```python
from build123d import *

# Parameters (mm, degrees)
BOSS_EXTRUDE1_START     = -2.5
BOSS_EXTRUDE1_OUTLINE_R = 2.075
BOSS_EXTRUDE1_DEPTH     = 5
FILLET1_R               = 10
FILLET2_R               = 2
SKETCH6_R               = 2.6
CUT_EXTRUDE3_DEPTH      = 0.6
CUT_EXTRUDE4_START      = -0.6
SKETCH7_R               = 2.6
CUT_EXTRUDE4_DEPTH      = 0.6


# Read off the part's stored shape, not the designer's step: Boss-Extrude1
with BuildPart() as part:
    # Boss-Extrude1 outline → Boss-Extrude1 (new body)
    with BuildSketch(Plane(origin=(0, 0, 0), x_dir=(0, 0, -1), z_dir=(1, 0, 0)).offset(BOSS_EXTRUDE1_START)):
        with BuildLine():
            add(Edge.make_bspline(
                [(-11.467759302, 5.348193827), (-9.897325632, 4.539306529), (-6.914913615, 3.521436488), (-2.263899905, 2.426855128), (2.06634335, 1.307705864), (6.2118215, -0.350082751), (10.140310372, -2.114581028), (13.169191833, -3.310542475), (14.923737301, -3.829233653), (15.372310037, -3.948537134)],
                knots=[0.083247791, 0.083247791, 0.083247791, 0.083247791, 0.25, 0.375, 0.5, 0.625, 0.75, 0.875, 0.917679059, 0.917679059, 0.917679059, 0.917679059], degree=3))
            ThreePointArc((-11.467759302, 5.348193827), (-17.179981816, 7.278246829), (-12.961908872, 2.969830498))
            add(Edge.make_bspline(
                [(-12.961908872, 2.969830498), (-12.439456061, 2.692527792), (-10.540790951, 1.792456097), (-7.150824595, 0.699411978), (-2.87827779, -0.304494056), (1.198988752, -1.360799538), (5.069797155, -2.90772863), (9.016006033, -4.678857357), (12.277896091, -5.971009628), (14.261338764, -6.553588571), (14.817570219, -6.697806322)],
                knots=[0.076895227, 0.076895227, 0.076895227, 0.076895227, 0.125, 0.25, 0.375, 0.5, 0.625, 0.75, 0.875, 0.922454156, 0.922454156, 0.922454156, 0.922454156], degree=3))
            ThreePointArc((14.817570219, -6.697806322), (20.84375711, -6.483151878), (15.372310037, -3.948537134))
        make_face()
        with Locations((17.805, -5.87)):
            Circle(BOSS_EXTRUDE1_OUTLINE_R, mode=Mode.SUBTRACT)
        with Locations((-14.555, 5.629165125)):
            Circle(BOSS_EXTRUDE1_OUTLINE_R, mode=Mode.SUBTRACT)
    extrude(amount=BOSS_EXTRUDE1_DEPTH)

    # Fillet1
    fillet1_edges = [part.edges().sort_by_distance(p)[0] for p in [
        (0, -6.697806322, -14.817570219),
        (0, 5.348193827, 11.467759302),
    ]]
    fillet(fillet1_edges, radius=FILLET1_R)

    # Fillet2
    fillet2_edges = [part.edges().sort_by_distance(p)[0] for p in [
        (0, -3.948537134, -15.372310037),
        (0, 2.969830498, 12.961908872),
    ]]
    fillet(fillet2_edges, radius=FILLET2_R)

    # Sketch6 → Cut-Extrude3 (cut)
    with BuildSketch(Plane(origin=(2.5, 0, 0), x_dir=(0, 0, -1), z_dir=(1, 0, 0))):
        with Locations((-14.555, 5.629165125)):
            Circle(SKETCH6_R)
        with Locations((17.805, -5.87)):
            Circle(SKETCH6_R)
    extrude(amount=-CUT_EXTRUDE3_DEPTH, mode=Mode.SUBTRACT)

    # Sketch7 → Cut-Extrude4 (cut)
    with BuildSketch(Plane.ZY.offset(2.5).offset(CUT_EXTRUDE4_START)):
        with Locations(Location((14.555, 5.629165125, 0), (0, 0, 180))):
            Circle(SKETCH7_R)
        with Locations(Location((-17.805, -5.87, 0), (0, 0, 180))):
            Circle(SKETCH7_R)
    extrude(amount=CUT_EXTRUDE4_DEPTH, mode=Mode.SUBTRACT)


solid = part.part
```
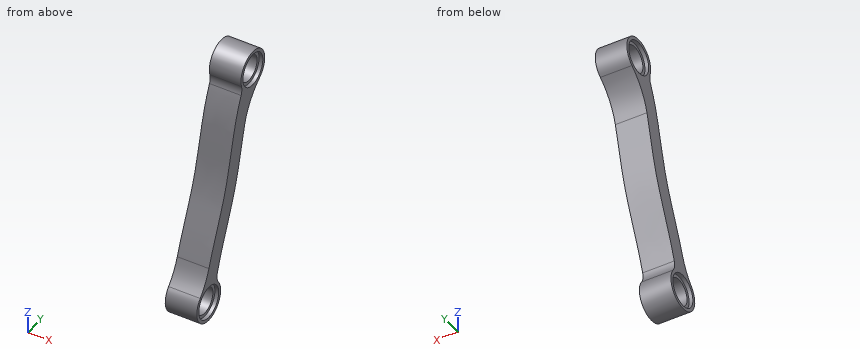
Geometry: final body of the model. Coordinates: model frame, mm. Coordinates: 2 decimals unless noted, no trailing zeros. Order: outer loops, then holes, each group sorted by start corner. A loop starts at its lowest first (then second) coordinate and runs counter-clockwise, first axis right, second up. Notation, with made-up numbers: (36.5, 44.5) - (77.5, 44.5) arc R21 cw to (77.5, 74.5) - close; hole circle Ø2 at (2.5, 86). An arc over 180 degrees is marked (long way). Return JSON: item names as keys, results as strings. Group by question number.
1. Material intervals for line 1 along Z through (x, y) = (-0.15, -7.75); line 2 along Z through (x, y) = (1.35, 4.75); line 3 along Y through (x, z) = (1.7, -3), sorted ascending. Write a range as [from, to].
2. Cut plane B-B (x = 1.4). Count the separate pieces of the cut face and the enclosed holes in it, plus the area to 3 significant figures.
3. Pin query (flat end, axial travel): pin 1 (4 mm diameter, centred on y = 5, z = 14.5, fed in from -X). Return the tip coordinate at first contact, or that it passes through.
4. Cut plane A-A (z = -18). Output: boundary loops of the cut face in (x, y).
Resolved:
{
 "1": {"line 1": "z = [-20.27, -18.68], [-16.93, -15.28]", "line 2": "z = [9.28, 12.68], [16.43, 17.53]", "line 3": "y = [-2.1, 0.89]"},
 "2": {"separate pieces": "1", "enclosed holes": "2", "area": "116 mm²"},
 "3": {"pin 1": "stops at x = -2.5"},
 "4": {"outline": "(-2.5, -8.96) - (2.5, -8.96) - (2.5, -8.46) - (1.9, -8.46) - (1.9, -7.94) - (-1.9, -7.94) - (-1.9, -8.46) - (-2.5, -8.46) - close; (-2.5, -3.28) - (-1.9, -3.28) - (-1.9, -3.8) - (1.9, -3.8) - (1.9, -3.28) - (2.5, -3.28) - (2.5, -2.78) - (-2.5, -2.78) - close"}
}
